The model under review builds one solid part; all positions refer to its coordinate system, in mm. A direction names the side the tool comes from. Round coordinates to 2 decimals unless told otherwise and drop trailing zeros. Loops run counter-clockwise (first coordinate to the right, second up) from the corner with the lowest first, then second, coordinate; pieces in that order, holes last. Notation, with made-up numbers: M 23,57.25 L 28,57.25 A22 cw 28,84.25 Z; hole C -17.75,55 d5. An arc over 180 degrees is marked long. Answer as a JSON object with one key per item and string values. Group by question number.
Item 1: Consider section A-A (x = 3). Give the boundary of the cut face in (y, z), and give its area (3 significant figures).
Item 2: The part is to be moulded in two halves that separate along X. For faces 1 (the face through (-14.2, 24.9, 27.8)), 2 (the face through (-1, -8, 0)), 3 (the face through (-32.11, -24.62, 24.65)), 4 (the face through (14.44, 24.76, 27.82)), say which applies: +X half, -X half, draft (parallel to the pull), parting line (faces both ways), or undercut.
Item 3: Consider section B-B (z = 28.5). Give the boundary of the cut face in (x, y).
Item 4: To check wall thickness, follow line 1 (Y direction, x = 0, z = 3.25); line 2 (Y direction, x = 12.5, z = 7); line 3 (Z direction, x = -5, y = -6.5). State the ranges of each line that lie inside material, in increasing order.
Item 5: Insertion check: P1, Ø2, axis at y = 10, z = 20.5, coming from the -X side; P2, Ø3, axis at x = 8.5, y = 9.5, coming from the +Z side; P3, Ø1.5, axis at y = 9, z = 7.5, coming from the -X side; P4, Ø9, axis at x = 0, y = 0, coming from the +Z side. Each pin has a flat end and moves straight along its axis. Give the tip position at first contact, or say it passes through.
Item 6: Consider section C-C (y = -1.5). Give the boundary of the cut face in (x, z), and give its area (3 significant figures).
Item 7: Tool access review of faces 5 (the face through (12, 27, 50)), 6 (the face through (0, -7, 5)): name each direction out of +Z, -Z, +X, -X, +Y, -Y from which nothing blocks a thin tool from reaching the whole face with its end or side.
Item 8: Consider section D-D (y = -12). Give the boundary of the cut face in (x, z).
```python
from build123d import *

# Parameters (mm, degrees)
F0_R     = 40.462362
F1_DEPTH = 50
F3_DEPTH = 45
F5_D     = 10


with BuildPart() as f1:
    # F0 (on Top) → F1 (new body)
    with BuildSketch(Plane.XY):
        Circle(F0_R)
    extrude(amount=F1_DEPTH)

    # F2 (on face) → F3 (cut)
    with BuildSketch(Plane.XY.offset(50)):
        Polygon((-0.125509, 33.096657), (-28.7253, 16.439635), (-28.599791, -16.657022), (0.125509, -33.096657), (28.7253, -16.439635), (28.599791, 16.657022), align=None)
    extrude(amount=-F3_DEPTH, mode=Mode.SUBTRACT)

    # F5 (through all)
    with Locations(Plane(origin=(0, 0, 0), x_dir=(1, 0, 0), z_dir=(0, 0, -1))):
        with Locations((0, 0)):
            Hole(F5_D / 2)


solid = f1.part
```
Geometry results:
{
 "1": {"outline": "M -40.35,0 L -4,0 L -4,5 L -31.42,5 L -31.42,50 L -40.35,50 Z; M 4,0 L 40.35,0 L 40.35,50 L 31.31,50 L 31.31,5 L 4,5 Z", "area": "1,170 mm^2"},
 "2": {"face 1": "undercut", "face 2": "draft", "face 3": "parting line", "face 4": "undercut"},
 "3": {"outline": "C 0,0 d80.92; hole M -28.73,16.44 L -28.6,-16.66 L 0.13,-33.1 L 28.73,-16.44 L 28.6,16.66 L -0.13,33.1 Z"},
 "4": {"line 1": "y = -40.46 to -5, 5 to 40.46", "line 2": "y = -38.48 to -25.89, 25.87 to 38.48", "line 3": "z = 0 to 5"},
 "5": {"P1": "stops at x = -39.45", "P2": "stops at z = 5", "P3": "stops at x = -39.61", "P4": "passes through"},
 "6": {"outline": "M -40.43,0 L -4.77,0 L -4.77,5 L -28.66,5 L -28.66,50 L -40.43,50 Z; M 4.77,0 L 40.43,0 L 40.43,50 L 28.67,50 L 28.67,5 L 4.77,5 Z", "area": "1,420 mm^2"},
 "7": {"face 5": "+Z, +X, -X, +Y, -Y", "face 6": "+Z"},
 "8": {"outline": "M -38.64,0 L 38.64,0 L 38.64,50 L 28.71,50 L 28.71,5 L -28.62,5 L -28.62,50 L -38.64,50 Z"}
}
